Read the model definition and answer for the solid it produces. Units are mm, in the model's axes. A direction names the side the tool comes from. Give positions to 0.01 mm unless a question says otherwise; leave off trailing zeros. Order: outer loops, then holes, each group sorted by start corner. A loop starts at its lowest first (then second) coordinate and runs counter-clockwise, first axis right, second up.
Item 1: Find the intervals of material crossed by line 1 along X through (y, z) = (21.5, 2.5); line 2 along Y through (x, z) = (-1.4, 18.5), in increasing order.
Item 2: A cutting plane is placed at C-C (y = 18.5). Write down the section's boundary in (x, z), plus the area to 3 significant figures.
Item 3: A cutting plane is placed at A-A (x = 16.75). Write down the section's boundary in (y, z).
Item 4: The mould has two halves that part along Z. Classify faces 1 (the face through (0.57, 0.6, 18.76)), 2 (the face through (9.34, -0.99, 1.8)), 3 (the face through (-1, 12, 0)): +Z half, -Z half, draft (parallel to the pull), parting line (faces both ways), or undercut.
Item 5: Given pin 1 Ø1 at (x, z) = (10, 31) entering from +Y; pin 2 Ø1 at (y, z) = (20.5, 9.5) entering from +X, each flat-ended and moving along its own axis, determine where each tip first touches the part or whether it passes through.
Item 6: A cutting plane is placed at B-B (z = 18.5). Write down the section's boundary in (x, y).
Item 7: Which of the six approach directions +Z, -Z, +X, -X, +Y, -Y give full straight-line access (tool end or side, diameter ignored) to faces 4 (the face through (10, -2, 18)), 5 (the face through (11, 0, 18))?
Item 8: A cutting plane is placed at D-D (z = 9). Write down the section's boundary in (x, y).
from build123d import *

# Parameters (mm, degrees)
BOSS_EXTRUDE1_DEPTH = 37
SKETCH2_R           = 6.5
SKETCH2_R_2         = 1.5
CUT_EXTRUDE1_DEPTH  = 10
SKETCH3_R           = 1.513801081
SKETCH3_R_2         = 1.495226131
CUT_EXTRUDE2_DEPTH  = 10
FILLET1_R           = 2
FILLET3_R           = 0.5
SKETCH5_W           = 7.144886566
SKETCH5_H           = 37
BOSS_EXTRUDE3_DEPTH = 2
SKETCH6_R           = 2.342689667
BOSS_EXTRUDE4_DEPTH = 2
FILLET5_R           = 2


with BuildPart() as part:
    # Sketch1 → Boss-Extrude1 (new body)
    with BuildSketch(Plane.XY):
        with BuildLine():
            Line((0, 0), (0, 37))
            Line((0, 37), (-2, 37))
            Line((-2, 37), (-2, -1))
            ThreePointArc((-2, -1), (-1.707106781, -1.707106781), (-1, -2))
            Line((-1, -2), (20.5, -2))
            Line((20.5, -2), (20.5, 0))
            Line((20.5, 0), (0, 0))
        make_face()
    extrude(amount=BOSS_EXTRUDE1_DEPTH)

    # Sketch2 → Cut-Extrude1 (cut)
    with BuildSketch(Plane(origin=(0, 0, 0), x_dir=(0, 0, -1), z_dir=(1, 0, 0))):
        with Locations((-18.5, 18.5)):
            Circle(SKETCH2_R)
        with Locations((-18.5, 9)):
            Circle(SKETCH2_R_2)
    extrude(amount=-CUT_EXTRUDE1_DEPTH, mode=Mode.SUBTRACT)

    # Sketch3 → Cut-Extrude2 (cut)
    with BuildSketch(Plane(origin=(0, 0, 0), x_dir=(1, 0, 0), z_dir=(0, 1, 0))):
        with Locations(Location((16.75, -2.987028894, 0), (0, 0, 270))):
            Circle(SKETCH3_R)
        with Locations(Location((10.25, -2.987028894, 0), (0, 0, 270))):
            Circle(SKETCH3_R_2)
        with Locations(Location((4, -2.987028894, 0), (0, 0, 270))):
            Circle(SKETCH3_R_2)
        with Locations(Location((16.75, -34.012971106, 0), (0, 0, 270))):
            Circle(SKETCH3_R)
        with Locations(Location((10.25, -34.012971106, 0), (0, 0, 270))):
            Circle(SKETCH3_R_2)
        with Locations(Location((4, -34.012971106, 0), (0, 0, 270))):
            Circle(SKETCH3_R_2)
    extrude(amount=-CUT_EXTRUDE2_DEPTH, mode=Mode.SUBTRACT)

    # Fillet1
    fillet1_edges = [part.edges().sort_by_distance(p)[0] for p in [
        (-1, 37, 37),
        (-1, 37, 0),
    ]]
    fillet(fillet1_edges, radius=FILLET1_R)

    # Fillet3
    fillet3_edges = [part.edges().sort_by_distance(p)[0] for p in [
        (20.5, -1, 37),
        (20.5, -1, 0),
    ]]
    fillet(fillet3_edges, radius=FILLET3_R)

    # Sketch5 → Boss-Extrude3 (add)
    with BuildSketch(Plane(origin=(0, 0, 0), x_dir=(1, 0, 0), z_dir=(0, 1, 0))):
        with Locations((3.572443283, -18.5)):
            Rectangle(SKETCH5_W, SKETCH5_H)
    extrude(amount=-BOSS_EXTRUDE3_DEPTH)

    # Sketch6 → Boss-Extrude4 (add)
    with BuildSketch(Plane(origin=(0, 0, 0), x_dir=(0, 0, -1), z_dir=(1, 0, 0))):
        with Locations((-18.5, 9)):
            Circle(SKETCH6_R)
    extrude(amount=-BOSS_EXTRUDE4_DEPTH)

    # Fillet5
    fillet5_edges = [part.edges().sort_by_distance(p)[0] for p in [
        (0, 0, 18.5),
    ]]
    fillet(fillet5_edges, radius=FILLET5_R)


solid = part.part
Response values:
1. line 1: x = -2 to 0
1. line 2: y = -1.92 to 12, 25 to 37
2. outline: (-2, 0) - (0, 0) - (0, 12) - (-2, 12) - close; (-2, 25) - (0, 25) - (0, 37) - (-2, 37) - close
2. area: 48.0 mm2
3. outline: (-2, 0) - (0, 0) - (0, 1.47) - (-2, 1.47) - close; (-2, 4.5) - (0, 4.5) - (0, 32.5) - (-2, 32.5) - close; (-2, 35.53) - (0, 35.53) - (0, 37) - (-2, 37) - close
4. face 1: draft
4. face 2: undercut
4. face 3: -Z half
5. pin 1: stops at y = 0
5. pin 2: stops at x = 0
6. outline: (-2, -1) arc R1 ccw to (-1, -2) - (20.5, -2) - (20.5, 0) - (2, 0) arc R2 cw to (0, 2) - (0, 12) - (-2, 12) - close; (-2, 25) - (0, 25) - (0, 37) - (-2, 37) - close
7. face 4: +Z, -Z, +X, -X, -Y
7. face 5: +Z, -Z, +X, +Y
8. outline: (-2, -1) arc R1 ccw to (-1, -2) - (20.5, -2) - (20.5, 0) - (2, 0) arc R2 cw to (0, 2) - (0, 37) - (-2, 37) - close
